The listing builds one solid part. Answer for the finished solid, in the listing's coordinates (mm). Face numbers are marked on the shaded views. A direction names the side the tool comes from. Round coordinates to 2 decimals unless told otherwise and drop trailing zeros. Loops run counter-clockwise (first coordinate to the right, second up) from the corner with the lowest first, then second, coordinate; pieces in that order, holes last. Notation, with made-up numbers: (72.25, -34) -> (111.25, -34) arc R11 cw to (111.25, -17) -> close; hole circle Ø5 at (-17, 39). An arc over 180 degrees is marked (long way). One line per question, with ' | ' between items.
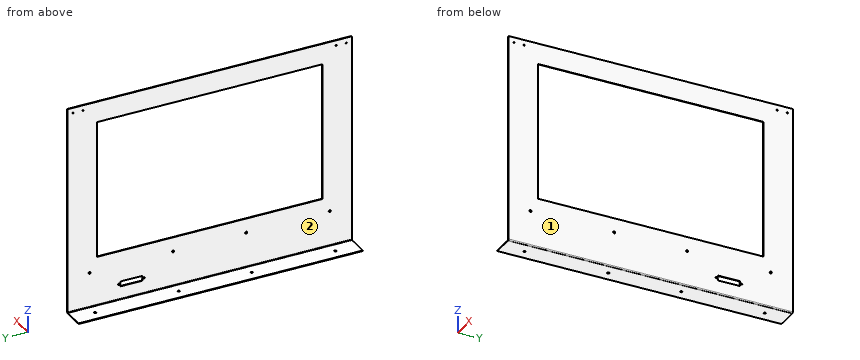
from build123d import *

# Parameters (mm, degrees)
SKETCH1_W                  = 680
SKETCH1_H                  = 550
SKETCH1_R                  = 1.5
BOSS_EXTRUDE1_DEPTH        = 1.3
SKETCH3_W                  = 540
SKETCH3_H                  = 330
CUT_EXTRUDE1_DEPTH         = 438.878125167
F_5_0_5_DIAMETER_HOLE1_D   = 5
CONVERT_SOLID1_START       = -0.2
CONVERT_SOLID1_OUTLINE_W   = 680
CONVERT_SOLID1_OUTLINE_H   = 550
CONVERT_SOLID1_OUTLINE_R   = 2.5
CONVERT_SOLID1_OUTLINE_R_2 = 1.5
CONVERT_SOLID1_OUTLINE_W_2 = 540
CONVERT_SOLID1_OUTLINE_H_2 = 330
CONVERT_SOLID1_DEPTH       = 0.2
SKETCHED_START             = -339.25
SKETCHED_BEND1_DEPTH       = 680
SKETCHED_BEND1_2_DEPTH     = 680
F_5_0_5_DIAMETER_HOLE2_D   = 5
CUT_EXTRUDE2_DEPTH         = 442.008177978
FILLET4_R                  = 1.5
FILLET5_R                  = 1.5
FILLET6_R                  = 1.5
FILLET7_R                  = 1.5
FILLET8_R                  = 1.5
FILLET9_R                  = 1.5
FILLET10_R                 = 1.5
FILLET11_R                 = 1.5


# Read off the part's stored shape, not the designer's step: Convert-Solid1, Sketched Bend1
with BuildPart() as part:
    # Sketch1 → Boss-Extrude1 (new body)
    with BuildSketch(Plane.YZ):
        with Locations((0.75, 0)):
            Rectangle(SKETCH1_W, SKETCH1_H)
        with Locations(Location((-326.141480577, 262.3, 0), (0, 0, 270))):
            Circle(SKETCH1_R, mode=Mode.SUBTRACT)
        with Locations(Location((-302.039034574, 262.3, 0), (0, 0, 270))):
            Circle(SKETCH1_R, mode=Mode.SUBTRACT)
        with Locations(Location((327.641480577, 262.3, 0), (0, 0, 270))):
            Circle(SKETCH1_R, mode=Mode.SUBTRACT)
        with Locations(Location((303.539034574, 262.3, 0), (0, 0, 270))):
            Circle(SKETCH1_R, mode=Mode.SUBTRACT)
    extrude(amount=BOSS_EXTRUDE1_DEPTH)

    # Sketch3 → Cut-Extrude1 (cut, through all)
    with BuildSketch(Plane.YZ.offset(1.3)):
        with Locations((0.75, 59.995312317)):
            Rectangle(SKETCH3_W, SKETCH3_H)
    extrude(amount=-CUT_EXTRUDE1_DEPTH, mode=Mode.SUBTRACT)

    # Ø5.0 (5) Diameter Hole1 (through all)
    with Locations(Plane.YZ.offset(1.3)):
        with Locations((288.05, -139.45), (-286.55, -139.45), (-86.55, -139.45), (88.05, -139.45)):
            Hole(F_5_0_5_DIAMETER_HOLE1_D / 2)

    # Convert-Solid1 outline → Convert-Solid1 (add)
    with BuildSketch(Plane.YZ.offset(CONVERT_SOLID1_START)):
        with Locations((0.75, 0)):
            Rectangle(CONVERT_SOLID1_OUTLINE_W, CONVERT_SOLID1_OUTLINE_H)
        with Locations((-286.55, -139.45)):
            Circle(CONVERT_SOLID1_OUTLINE_R, mode=Mode.SUBTRACT)
        with Locations((-86.55, -139.45)):
            Circle(CONVERT_SOLID1_OUTLINE_R, mode=Mode.SUBTRACT)
        with Locations((88.05, -139.45)):
            Circle(CONVERT_SOLID1_OUTLINE_R, mode=Mode.SUBTRACT)
        with Locations((288.05, -139.45)):
            Circle(CONVERT_SOLID1_OUTLINE_R, mode=Mode.SUBTRACT)
        with Locations((-326.141480577, 262.3)):
            Circle(CONVERT_SOLID1_OUTLINE_R_2, mode=Mode.SUBTRACT)
        with Locations((-302.039034574, 262.3)):
            Circle(CONVERT_SOLID1_OUTLINE_R_2, mode=Mode.SUBTRACT)
        with Locations((0.75, 59.995312317)):
            Rectangle(CONVERT_SOLID1_OUTLINE_W_2, CONVERT_SOLID1_OUTLINE_H_2, mode=Mode.SUBTRACT)
        with Locations((303.539034574, 262.3)):
            Circle(CONVERT_SOLID1_OUTLINE_R_2, mode=Mode.SUBTRACT)
        with Locations((327.641480577, 262.3)):
            Circle(CONVERT_SOLID1_OUTLINE_R_2, mode=Mode.SUBTRACT)
    extrude(amount=CONVERT_SOLID1_DEPTH)

    # Sketched Bend1 outline → Sketched Bend1 (cut)
    with BuildSketch(Plane(origin=(0, 0, 0), x_dir=(1, 0, 0), z_dir=(0, 1, 0)).offset(SKETCHED_START)):
        with BuildLine():
            Line((-0.2, 275), (-0.2, 224.598076212))
            ThreePointArc((-0.2, 224.598076212), (0.898076212, 223.5), (1.3, 222))
            Line((1.3, 222), (1.3, 275))
            Line((1.3, 275), (-0.2, 275))
        make_face()
    extrude(amount=SKETCHED_BEND1_DEPTH, mode=Mode.SUBTRACT)

    # Sketched Bend1 2 outline → Sketched Bend1 2 (add)
    with BuildSketch(Plane(origin=(0, 0, 0), x_dir=(1, 0, 0), z_dir=(0, 1, 0)).offset(SKETCHED_START)):
        with BuildLine():
            Line((-51.165708265, 225), (-51.165708265, 223.5))
            Line((-51.165708265, 223.5), (-1.7, 223.5))
            ThreePointArc((-1.7, 223.5), (-0.639339828, 223.060660172), (-0.2, 222))
            Line((-0.2, 222), (-0.2, 224.598076212))
            ThreePointArc((-0.2, 224.598076212), (-0.923542865, 224.897777479), (-1.7, 225))
            Line((-1.7, 225), (-51.165708265, 225))
        make_face()
    extrude(amount=SKETCHED_BEND1_2_DEPTH)

    # Ø5.0 (5) Diameter Hole2 (through all)
    with Locations(Plane(origin=(0, 0, -223.5), x_dir=(0, -1, 0), z_dir=(0, 0, 1))):
        with Locations((-288.05, -26.165708265), (-88.05, -26.165708265), (86.55, -26.165708265), (286.55, -26.165708265)):
            Hole(F_5_0_5_DIAMETER_HOLE2_D / 2)

    # Sketch15 → Cut-Extrude2 (cut, through all)
    with BuildSketch(Plane.YZ.offset(1.3)):
        Polygon((161.5, -180), (214.6, -180), (214.6, -184.45), (220.1, -184.45), (220.1, -187.55), (214.6, -187.55), (214.6, -192), (161.5, -192), (161.5, -187.55), (156, -187.55), (156, -184.45), (161.5, -184.45), align=None)
    extrude(amount=-CUT_EXTRUDE2_DEPTH, mode=Mode.SUBTRACT)

    # Fillet4
    fillet4_edges = [part.edges().sort_by_distance(p)[0] for p in [
        (0.55, 161.5, -180),
    ]]
    fillet(fillet4_edges, radius=FILLET4_R)

    # Fillet5
    fillet5_edges = [part.edges().sort_by_distance(p)[0] for p in [
        (0.55, 214.6, -180),
    ]]
    fillet(fillet5_edges, radius=FILLET5_R)

    # Fillet6
    fillet6_edges = [part.edges().sort_by_distance(p)[0] for p in [
        (0.55, 220.1, -184.45),
    ]]
    fillet(fillet6_edges, radius=FILLET6_R)

    # Fillet7
    fillet7_edges = [part.edges().sort_by_distance(p)[0] for p in [
        (0.55, 220.1, -187.55),
    ]]
    fillet(fillet7_edges, radius=FILLET7_R)

    # Fillet8
    fillet8_edges = [part.edges().sort_by_distance(p)[0] for p in [
        (0.55, 214.6, -192),
    ]]
    fillet(fillet8_edges, radius=FILLET8_R)

    # Fillet9
    fillet9_edges = [part.edges().sort_by_distance(p)[0] for p in [
        (0.55, 161.5, -192),
    ]]
    fillet(fillet9_edges, radius=FILLET9_R)

    # Fillet10
    fillet10_edges = [part.edges().sort_by_distance(p)[0] for p in [
        (0.55, 156, -184.45),
    ]]
    fillet(fillet10_edges, radius=FILLET10_R)

    # Fillet11
    fillet11_edges = [part.edges().sort_by_distance(p)[0] for p in [
        (0.55, 156, -187.55),
    ]]
    fillet(fillet11_edges, radius=FILLET11_R)


solid = part.part
Q1. For the marked faces 1 and 2, determine the directions among +Z, -Z, +X, -X, +Y, -Y from which every point of the face is accessible in a straight line to the end or side of a thin tool.
Numbers:
face 1: +Z, -Z, +X, +Y, -Y | face 2: +Z, -X, +Y, -Y
Q2. Find the intervals of material crossed by line 1 (Z direction, x = -0.05, y = -86.55); line 2 (Y direction, x = 0.5, z = -139.45); line 3 (Y direction, x = 0, z = 262), in increasing order. Write a range as from..to.
Numbers:
line 1: -224.51..-141.95, -136.95..-105, 225..275 | line 2: -339.25..-289.05, -284.05..-89.05, -84.05..85.55, 90.55..285.55, 290.55..340.75 | line 3: -339.25..-327.61, -324.67..-303.51, -300.57..302.07, 305.01..326.17, 329.11..340.75
Q3. Given pin 1 Ø6.5 at (y, z) = (88.05, -139.45) entering from +X; pin 2 Ø5 at (x, y) = (-22, 18) entering from +Z; pin 3 Ø0.8 at (x, y) = (0.5, 198) entering from -Z; pin 4 Ø0.8 at (x, y) = (0, 160) entering from -Z, each flat-ended and moving along its own axis, determine where each tip first touches the part or whether it passes through.
Numbers:
pin 1: x = 1.3 | pin 2: z = -223.5 | pin 3: z = -224.4 | pin 4: z = -224.7
Q4. A cutting plane is placed at D-D on z = -125. Give the vertices of the cut face in (x, y), plus the area to 3 significant figures.
Numbers:
outline: (-0.2, -339.25) -> (1.3, -339.25) -> (1.3, 340.75) -> (-0.2, 340.75) -> close | area: 1,020 mm^2
Q5. A cutting plane is placed at C-C on y = -233. Give the vertices of the cut face in (x, z), plus the area to 3 significant figures.
Numbers:
outline: (-51.17, -225) -> (-1.7, -225) arc R3 ccw to (1.3, -222) -> (1.3, -105) -> (-0.2, -105) -> (-0.2, -222) arc R1.5 cw to (-1.7, -223.5) -> (-51.17, -223.5) -> close; (-0.2, 225) -> (1.3, 225) -> (1.3, 275) -> (-0.2, 275) -> close | area: 330 mm^2
Q6. A cutting plane is placed at B-B on y = 178. Give the vertices of the cut face in (x, z), plus the area to 3 significant figures.
Numbers:
outline: (-51.17, -225) -> (-1.7, -225) arc R3 ccw to (1.3, -222) -> (1.3, -192) -> (-0.2, -192) -> (-0.2, -222) arc R1.5 cw to (-1.7, -223.5) -> (-51.17, -223.5) -> close; (-0.2, -180) -> (1.3, -180) -> (1.3, -105) -> (-0.2, -105) -> close; (-0.2, 225) -> (1.3, 225) -> (1.3, 275) -> (-0.2, 275) -> close | area: 312 mm^2
Q7. A cutting plane is placed at A-A on z = 50. Give the vertices of the cut face in (x, y).
Numbers:
outline: (-0.2, -339.25) -> (1.3, -339.25) -> (1.3, -269.25) -> (-0.2, -269.25) -> close; (-0.2, 270.75) -> (1.3, 270.75) -> (1.3, 340.75) -> (-0.2, 340.75) -> close
